Read the model definition and answer for the solid it produces. Units are mm, in the model's axes. A direction names the side the tool comes from. Coordinates: 2 decimals unless noted, no trailing zeros. Loops run counter-clockwise (first coordinate to the right, second up) from the corner with the lowest first, then second, coordinate; pieces in that order, holes last. Notation, with made-up numbers: (30, 34.25) - (83, 34.25) arc R15 ccw to (83, 63.25) - close; hole circle Ø3 at (74.25, 28.25). An arc over 180 degrees is marked (long way). One line per item, written item: value. Start each with the question number.
Autodesk Inventor part; units mm, degrees
ref_plane "YZ Plane" through (0, 0, 0) normal (1, 0, 0) x (0, 1, 0)
ref_plane "XZ Plane" through (0, 0, 0) normal (0, 1, 0) x (-1, 0, 0)
ref_plane "XY Plane" through (0, 0, 0) normal (0, 0, 1) x (1, 0, 0)
sketch "Sketch1" plane through (0, 0, 0) normal (0, 1, 0) x (-1, 0, 0)
  line L0 (0, -1.778) -> (2.413, -1.778)
  line L1 (2.413, -1.778) -> (2.413, -10.16)
  line L2 (2.413, -10.16) -> (3.175, -10.16)
  line L3 (3.175, -10.16) -> (3.175, -11.43)
  line L4 (3.175, -11.43) -> (3.683, -11.43)
  line L5 (3.683, -11.43) -> (3.683, -2.032)
  line L6 (3.683, -2.032) -> (4.953, -2.032)
  line L7 (4.953, -2.032) -> (4.953, -0.254)
  line L8 (0, -0.254) -> (0, -1.778)
  line L9 (0, -0.254) -> (2.413, -0.254)
  line L10 (2.413, -0.254) -> (2.413, 4.572)
  line L11 (2.413, 4.572) -> (3.175, 4.572)
  line L12 (3.175, 4.572) -> (3.175, 10.922)
  line L13 (3.175, 10.922) -> (3.81, 10.922)
  line L14 (3.81, 10.922) -> (3.81, 9.652)
  line L15 (4.953, -0.254) -> (3.683, -0.254)
  line L16 (3.683, -0.254) -> (3.429, -0.254)
  line L17 (3.556, -0.254) -> (3.429, 9.652)
  line L18 (3.81, 9.652) -> (3.429, 9.652)
  line L19 (0, 10.922) -> (0, -12.4282) construction
  point P0 (0, 0)
  dimension "d0" = 1.778
  dimension "d1" = 2.413
  dimension "d2" = 8.382
  dimension "d3" = 0.762
  dimension "d4" = 1.27
  dimension "d5" = 0.508
  dimension "d6" = 9.398
  dimension "d7" = 1.27
  dimension "d8" = 1.778
  dimension "d9" = 4.826
  dimension "d10" = 0.762
  dimension "d11" = 6.35
  dimension "d12" = 0.635
  dimension "d13" = 1.27
  dimension "d14" = 1.27
  dimension "d15" = 0.254
revolve "Revolution1" add sketch "Sketch1" angle 360 about axis through (0, 0, 10.922) along (0, 0, -1)
sketch "Sketch2" plane through (0, 0, 10.922) normal (0, 0, 1) x (1, 0, 0)
  circle A0 centre (0, 0) radius 3.81
  line L0 (0, 3.81) -> (0.508, 3.81)
  line L1 (0, 3.81) -> (0.508, 3.81) construction
  line L2 (0.508, 3.81) -> (0.508, 2.9079)
  line L3 (0.508, 2.9079) -> (-0.508, 2.9079)
  line L4 (-0.508, 2.9079) -> (-0.508, 3.81)
  line L5 (-0.508, 3.81) -> (0, 3.81)
  line L6 (-0.508, -2.9079) -> (0.508, -2.9079)
  line L7 (0.508, -2.9079) -> (0.508, -3.81)
  line L8 (-0.508, -3.81) -> (-0.508, -2.9079)
  line L9 (0.508, -3.81) -> (0, -3.81)
  point P0 (-0.508, -3.776)
  point P1 (0.508, -3.776)
  point P2 (0.508, 3.776)
  point P3 (-0.508, 3.776)
  dimension "d17" = 0.508
  dimension "d18" = 0
  dimension "d19" = 1.016
  dimension "d22" = 360
extrude "Extrusion1" cut sketch "Sketch2" against normal blind 5.08 contours L2 L3 L4 A0 | A0 L8 L6 L7
properties part number "AxleGBR"
1) For faces 4 (the cylindrical face through (1.915, 1.468, 2.193)), 5 (the flat face through (0, 4, -2.032)), 6 (the flat face through (-3.6, -0.3, 9.652)), determine the directions among +Z, -Z, +X, -X, +Y, -Y from which every point of the face is accessible in a straight line to the end or side of a thin tool.
2) Straight lines are drawn through the part: L1, parallel to Y at x = 0, z = -10.75 (3 decimals); L2, parallel to Z at x = 0, y = -1; L3, parallel to Z at x = 3.75, y = -1.5. For each, find the intervals that lie inside material, in ascending order.
3) Determine the mould class of faces 1 (the conical face through (0.8, -3.4, 4.6)), 2 (the flat face through (-3.3, -0.5, 10.922)), 3 (the cylindrical face through (-3.81, -0.08, 10.28)) for opening direction Z: released by +Z, released by -Z, zero draft, split by the parting line, or undercut.
4) Section C-C, the plane y = 4.25 is taken. Determine the outline of the cut face in (x, z), and give its area (3 significant figures).
5) Section A-A, the plane z = 8.25 is taken. Determine the outline of the cut face in (x, y) (3 decimals).
6) Section B-B, the plane z = -4.75 is taken. Determine the outline of the cut face in (x, y).
7) Section D-D, the plane z = 1.5 is taken. Determine the outline of the cut face in (x, y), and give its area (3 significant figures).
8) Flat-ended cylindrical pins translate along their axes: P1, Ø4, axis at x = 0, y = 0, coming from the +Z side; P2, Ø2, axis at x = -2, z = 1, coming from the -Y side; P3, Ø3, axis at x = 0, y = -1, coming from the -Z side; P4, Ø1, axis at x = -3, y = 2.5, coming from the -Z side. Find the tip coordinate at first contact, or state that the pin passes through.
Answer below:
1. face 4: +Z
1. face 5: -Z
1. face 6: -X
2. L1: -3.683 to -3.175, 3.175 to 3.683
2. L2: -1.78 to -0.25
2. L3: -2.03 to -0.25
3. face 1: undercut
3. face 2: released by +Z
3. face 3: zero draft
4. outline: (-2.54, -2.03) - (2.54, -2.03) - (2.54, -0.25) - (-2.54, -0.25) - close
4. area: 9.04 mm2
5. outline: (-0.508, -3.409) - (-0.508, -3.134) arc R3.175 cw to (-0.508, 3.134) - (-0.508, 3.409) arc R3.447 ccw to start; (0.508, -3.409) arc R3.447 ccw to (0.508, 3.409) - (0.508, 3.134) arc R3.175 cw to (0.508, -3.134) - close
6. outline: circle Ø7.37 at (0, 0); hole circle Ø4.83 at (0, 0)
7. outline: circle Ø7.07 at (0, 0); hole circle Ø4.83 at (0, 0)
7. area: 20.9 mm2
8. P1: z = -0.25
8. P2: y = -3.4
8. P3: z = -10.16
8. P4: z = -11.43
